The listing builds one solid part. Answer for the finished solid, in the listing's coordinates (mm). A direction names the side the tool comes from. Round coordinates to 2 decimals unless told otherwise and drop trailing zeros. Write each loop counter-clockwise with the first axis right and the second up, starting at its lowest first coordinate (ties: lowest second). Pieces come first, ordered by that corner, then holes. Notation, with made-up numbers: M -9.75,23.25 L 15.25,23.25 A30 cw 15.25,50.25 Z; hole C -28.75,34.25 d8. An arc over 180 degrees is marked long. One line per item, written item: value. Start each with the question number.
(1) Section B-B (x = 11) is taken. Determine the outline of the cut face in (y, z), plus the area to 3 significant figures.
(2) Section A-A (z = 18.5) is taken. Determine the outline of the cut face in (x, y).
(3) Section D-D (y = 0) is taken. State how many separate pieces and enclosed holes the cut face has, plus the area to 3 significant figures.
(4) Given P1, Ø3.5, axis at x = 15.5, z = 18.5, coming from the -Y side; P2, Ø0.5, axis at y = -2.5, z = 13.5, coming from the +X side; P3, Ø2.5, axis at y = -4, z = 19.5, coming from the +X side, each flat-ended and moving along its own axis, determine where each tip first touches the part or whether it passes through.
(5) For a pull along Z with two mould halves and no side action, classify faces 1 (the flat face through (-14, 8.69, 17)), 2 (the flat face through (-14, -11.073, 18)), 3 (the flat face through (-14, 0, 22)) as released by +Z, released by -Z, zero draft, split by the parting line, or undercut.
(6) Section C-C (x = 1.5) is taken. Determine the outline of the cut face in (y, z), plus the area to 3 significant figures.
(7) For faces 4 (the flat face through (14, -8.414, 17)), 5 (the flat face through (14, -10.946, 18)), 6 (the flat face through (17.172, 0, 20)), 7 (the flat face through (22.7, 0.1, 3)), determine the directions among +Z, -Z, +X, -X, +Y, -Y from which every point of the face is accessible in a straight line to the end or side of a thin tool.
(8) Consider probe 1 along Z at (x, y) = (10, -3.5); probe 2 along X at (y, z) = (-4.75, 12.5); probe 3 along Y at (x, z) = (19, 10). Determine where each line is inside the solid, lowest interval first.
```python
from build123d import *

# Parameters (mm, degrees)
SKETCH_W        = 60
SKETCH_H        = 20
PAD_DEPTH       = 3
SKETCH001_W     = 40
SKETCH001_H     = 20
PAD001_DEPTH    = 10
SKETCH002_W     = 42
SKETCH002_H     = 22
PAD002_DEPTH    = 1
SKETCH003_W     = 7.210509
SKETCH003_H     = 22.018964
PAD003_DEPTH    = 8
SKETCH010_W     = 17.104093
SKETCH010_H     = 5.482681
POCKET_DEPTH    = 40
POCKET001_DEPTH = 5
SKETCH012_R     = 2.5
POCKET002_DEPTH = 5


with BuildPart() as part:
    # Sketch → Pad (new body)
    with BuildSketch(Plane.XY):
        Rectangle(SKETCH_W, SKETCH_H)
    extrude(amount=PAD_DEPTH)

    # Sketch001 (on Face6 of Pad) → Pad001 (join)
    with BuildSketch(Plane.XY.offset(3)):
        Rectangle(SKETCH001_W, SKETCH001_H)
    extrude(amount=PAD001_DEPTH)

    # Sketch002 → Pad002 (join)
    with BuildSketch(Plane.XY.offset(13)):
        Rectangle(SKETCH002_W, SKETCH002_H)
    extrude(amount=PAD002_DEPTH)

    # Sketch003 (on Face15 of Pad002) → Pad003 (join)
    with BuildSketch(Plane.XY.offset(14)):
        with Locations((-13.566278, -0.063386)):
            Rectangle(SKETCH003_W, SKETCH003_H)
        with Locations((13.566278, 0.063386)):
            Rectangle(SKETCH003_W, SKETCH003_H)
    extrude(amount=PAD003_DEPTH)

    # Sketch010 (on Face21 of Pad003) → Pocket (cut, symmetric)
    with BuildSketch(Plane.YZ.offset(-9.961024)):
        with Locations((0.137935, 16.812696)):
            Rectangle(SKETCH010_W, SKETCH010_H)
    extrude(amount=POCKET_DEPTH, both=True, mode=Mode.SUBTRACT)

    # Sketch011 (on Face10 of Pocket) → Pocket001 (cut)
    with BuildSketch(Plane.XY.offset(3)):
        with BuildLine():
            ThreePointArc((-26.414192, 10.338834), (-29.320565, 8.950898), (-30.662811, 6.023143))
            Line((-30.662811, 6.023143), (-30.662811, 10.298891))
            Line((-30.662811, 10.298891), (-26.414192, 10.338834))
        make_face()
        with BuildLine():
            ThreePointArc((-30.662811, -6.023143), (-29.320565, -8.950898), (-26.414192, -10.338834))
            Line((-30.662811, -10.298891), (-26.414192, -10.338834))
            Line((-30.662811, -6.023143), (-30.662811, -10.298891))
        make_face()
        with BuildLine():
            ThreePointArc((30.662811, 6.023143), (29.320565, 8.950898), (26.414192, 10.338834))
            Line((30.662811, 10.298891), (26.414192, 10.338834))
            Line((30.662811, 6.023143), (30.662811, 10.298891))
        make_face()
        with BuildLine():
            ThreePointArc((26.414192, -10.338834), (29.320565, -8.950898), (30.662811, -6.023143))
            Line((30.662811, -6.023143), (30.662811, -10.298891))
            Line((30.662811, -10.298891), (26.414192, -10.338834))
        make_face()
    extrude(amount=-POCKET001_DEPTH, mode=Mode.SUBTRACT)

    # Sketch012 (on Face12 of Pocket001) → Pocket002 (cut)
    with BuildSketch(Plane.XY.offset(3)):
        with Locations((-25.503695, 0)):
            Circle(SKETCH012_R)
        with Locations((25.497604, 0)):
            Circle(SKETCH012_R)
    extrude(amount=-POCKET002_DEPTH, mode=Mode.SUBTRACT)


solid = part.part
```
Recorded:
1. outline: M -11,13 L -10,13 L -10,0 L 10,0 L 10,13 L 11,13 L 11,14 L 11.07,14 L 11.07,22 L -10.95,22 L -10.95,14 L -11,14 Z; hole M -8.41,14.07 L 8.69,14.07 L 8.69,19.55 L -8.41,19.55 Z
1. area: 364 mm2
2. outline: M -17.17,-11.07 L -9.96,-11.07 L -9.96,-8.41 L -17.17,-8.41 Z; M -17.17,8.69 L -9.96,8.69 L -9.96,10.95 L -17.17,10.95 Z; M 9.96,-10.95 L 17.17,-10.95 L 17.17,-8.41 L 9.96,-8.41 Z; M 9.96,8.69 L 17.17,8.69 L 17.17,11.07 L 9.96,11.07 Z
3. separate pieces: 5
3. enclosed holes: 0
3. area: 628 mm2
4. P1: stops at y = -10.95
4. P2: stops at x = 21
4. P3: stops at x = 17.17
5. face 1: undercut
5. face 2: zero draft
5. face 3: released by +Z
6. outline: M -11,13 L -10,13 L -10,0 L 10,0 L 10,13 L 11,13 L 11,14 L -11,14 Z
6. area: 282 mm2
7. face 4: +X, -X
7. face 5: +Z, +X, -Y
7. face 6: +Z, +X, +Y, -Y
7. face 7: +X, +Y, -Y
8. probe 1: z = 0 to 14.07, 19.55 to 22
8. probe 2: x = -20 to 20
8. probe 3: y = -10 to 10
